```python
from build123d import *

# Parameters (mm, degrees)
F0_R     = 11.151047
F1_DEPTH = 25.4


with BuildPart() as f1:
    # F0 (on Front) → F1 (new body)
    with BuildSketch(Plane.XZ):
        with BuildLine():
            ThreePointArc((6.467178, -27.833545), (22.375547, -17.772605), (28.575, 0))
            ThreePointArc((28.575, 0), (23.076019, 16.853129), (8.695527, 27.219817))
            ThreePointArc((8.695527, 27.219817), (-28.551621, 1.15566), (6.467178, -27.833545))
        make_face()
        with BuildLine():
            ThreePointArc((-9.006877, 6.574345), (0, 11.151047), (9.006877, 6.574345))
            Line((9.006877, 6.574345), (20.940501, 6.574345))
            Line((20.940501, 6.574345), (20.940501, -6.574345))
            Line((20.940501, -6.574345), (9.006877, -6.574345))
            ThreePointArc((9.006877, -6.574345), (0, -11.151047), (-9.006877, -6.574345))
            Line((-9.006877, -6.574345), (-20.940501, -6.574345))
            Line((-20.940501, -6.574345), (-20.940501, 6.574345))
            Line((-20.940501, 6.574345), (-9.006877, 6.574345))
        make_face(mode=Mode.SUBTRACT)
        with BuildLine():
            ThreePointArc((-9.006877, -6.574345), (-11.151047, 0), (-9.006877, 6.574345))
            Line((-9.006877, 6.574345), (-20.940501, 6.574345))
            Line((-20.940501, 6.574345), (-20.940501, -6.574345))
            Line((-20.940501, -6.574345), (-9.006877, -6.574345))
        make_face()
        with BuildLine():
            ThreePointArc((8.695527, 27.219817), (23.076019, 16.853129), (28.575, 0))
            ThreePointArc((28.575, 0), (22.375547, -17.772605), (6.467178, -27.833545))
            Line((6.467178, -27.833545), (52.769401, -19.011813))
            ThreePointArc((52.769401, -19.011813), (34.925403, -0.123852), (52.522301, 18.99453))
            Line((52.522301, 18.99453), (8.695527, 27.219817))
        make_face()
        with BuildLine():
            ThreePointArc((73.025, 0), (66.921594, 13.974556), (52.522301, 18.99453))
            ThreePointArc((52.522301, 18.99453), (34.925403, -0.123852), (52.769401, -19.011813))
            ThreePointArc((52.769401, -19.011813), (67.012174, -13.890089), (73.025, 0))
        make_face()
        with Locations((53.975, 0)):
            Circle(F0_R, mode=Mode.SUBTRACT)
    extrude(amount=F1_DEPTH)


solid = f1.part
```
Read the model definition and answer for the solid it produces. Units are mm, in the model's axes. A direction names the side the tool comes from. Coordinates: 2 decimals unless noted, no trailing zeros. Order: outer loops, then holes, each group sorted by start corner. A loop starts at its lowest first (then second) coordinate and runs counter-clockwise, first axis right, second up. Notation, with made-up numbers: (43, 43) - (97, 43) arc R5 cw to (97, 51) - close; hole circle Ø1 at (80, 4.5). An arc over 180 degrees is marked (long way). Answer as a JSON object with one key per item and string values. Group by question number.
Item 1: Section A-A (x = 0) is taken. Give the vertices of the cut face in (y, z) (3 decimals), plus the area to 3 significant figures.
Item 2: Section D-D (x = 61.5) is taken. Give the vertices of the cut face in (y, z), plus the area to 3 significant figures.
Item 3: The mould has two halves that part along X. Classify faces 3 (the face through (-28.512, -12.522, 1.891)), 4 (the face through (22, -25.4, 0)), 5 (the face through (15, -13, -6.574)): +X half, -X half, draft (parallel to the pull), parting line (faces both ways), or undercut.
Item 4: Section B-B (y = -21.5) is taken. State how many separate pieces and enclosed holes the cut face has, plus the area to 3 significant figures.
Item 5: Consider probe 1 along X at (y, z) = (-23.5, 2); probe 2 along X at (y, z) = (-21.75, -10); probe 3 along Z at (x, y) = (57, -11). Determine where each line is inside the solid, lowest interval first. Write a range as from..to.
Item 6: A tool of negligible diameter and unlimited length cuts with its end or side. For faces 1 (the face through (20.941, -13, 0)), 2 (the face through (22, 0, 0)), from which of +Z, -Z, +X, -X, +Y, -Y can it reach the whole face along a straight path? Write none if from no direction.
Item 7: Flat-ended cylindrical pins translate along their axes: P1, Ø3, axis at x = 7.5, y = -7.5, coming from the +Z side; P2, Ø9.5, axis at x = 16, y = -18, coming from the +Z side; P3, Ø3.5, axis at x = 12, y = -11.5, coming from the -Z side. Find the tip coordinate at first contact, or state that the pin passes through.
Item 8: Section C-C (z = 5) is taken. Give the vertices of the cut face in (x, y), plus the area to 3 significant figures.
Results are:
{
 "1": {"outline": "(-25.4, -28.575) - (0, -28.575) - (0, -11.151) - (-25.4, -11.151) - close; (-25.4, 11.151) - (0, 11.151) - (0, 28.575) - (-25.4, 28.575) - close", "area": "885 mm^2"},
 "2": {"outline": "(-25.4, -17.5) - (0, -17.5) - (0, -8.23) - (-25.4, -8.23) - close; (-25.4, 8.23) - (0, 8.23) - (0, 17.5) - (-25.4, 17.5) - close", "area": "471 mm^2"},
 "3": {"face 3": "parting line", "face 4": "draft", "face 5": "undercut"},
 "4": {"separate pieces": "1", "enclosed holes": "2", "area": "3,510 mm^2"},
 "5": {"probe 1": "x = -28.5..-10.97, 20.94..43, 64.95..72.92", "probe 2": "x = -26.77..-4.93, 4.93..49.04, 58.91..70.19", "probe 3": "z = -18.81..-10.73, 10.73..18.81"},
 "6": {"face 1": "+Y, -Y", "face 2": "+Z, -Z, +X, -X, +Y"},
 "7": {"P1": "stops at z = 27.94", "P2": "stops at z = 26.74", "P3": "stops at z = -27.11"},
 "8": {"outline": "(-28.13, -25.4) - (-9.97, -25.4) - (-9.97, 0) - (-28.13, 0) - close; (20.94, -25.4) - (44.01, -25.4) - (44.01, 0) - (20.94, 0) - close; (63.94, -25.4) - (72.36, -25.4) - (72.36, 0) - (63.94, 0) - close", "area": "1,260 mm^2"}
}
